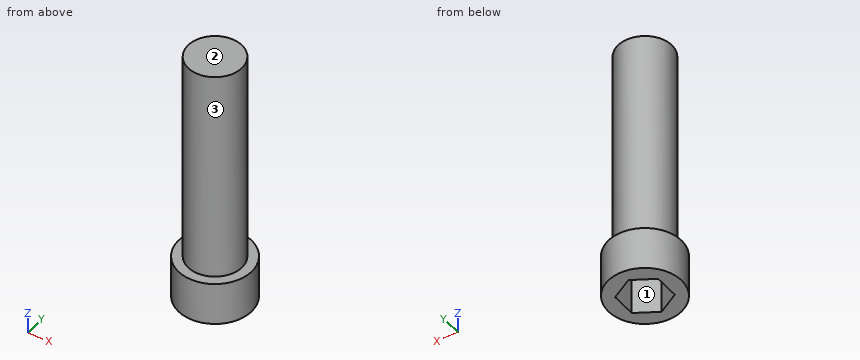
```python
from build123d import *

# Parameters (mm, degrees)
SKETCH1_R           = 1.25
BOSS_EXTRUDE1_DEPTH = 12
SKETCH1_3_R         = 1.7
SKETCH1_3_R_2       = 1.25
BOSS_EXTRUDE2_DEPTH = 2
CUT_EXTRUDE1_DEPTH  = 2


with BuildPart() as part:
    # Sketch1 → Boss-Extrude1 (new body)
    with BuildSketch(Plane.XY):
        Circle(SKETCH1_R)
    extrude(amount=BOSS_EXTRUDE1_DEPTH)

    # Sketch1<3> → Boss-Extrude2 (add)
    with BuildSketch(Plane.XY):
        Circle(SKETCH1_3_R)
        Circle(SKETCH1_3_R_2, mode=Mode.SUBTRACT)
    extrude(amount=BOSS_EXTRUDE2_DEPTH)

    # Sketch3 → Cut-Extrude1 (cut)
    with BuildSketch(Plane(origin=(0, 0, 0), x_dir=(-1, 0, 0), z_dir=(0, 0, -1))):
        Polygon((0.988114182, -0.597464389), (1.01147643, 0.556999789), (0.023362248, 1.154464178), (-0.988114182, 0.597464389), (-1.01147643, -0.556999789), (-0.023362248, -1.154464178), align=None)
    extrude(amount=-CUT_EXTRUDE1_DEPTH, mode=Mode.SUBTRACT)


solid = part.part
```
Can you work these out from the model? Positions are in its coordinate system, mm. Face numbers are marked on the shaded views. Round coordinates to 2 decimals unless told otherwise and drop trailing zeros. Loops run counter-clockwise (first coordinate to the right, second up) from the corner with the lowest first, then second, coordinate; pieces in that order, holes last. Notation, with made-up numbers: (24, 45) -> (41, 45) arc R9 ccw to (41, 61) -> close; hole circle Ø1 at (25, -1). An arc over 180 degrees is marked (long way). One line per item, written item: value. Start each with the question number.
1. If we mould it in two halves opening along Y, with no side actions, what happens to the marked faces 1, 2 and 3? For each: pulls with the +Y half, pulls with the -Y half, needs draft (parallel to the pull), parting line crosses it, or undercut.
2. If I drill on probe 1 along Z at (x, y) = (0.2, 0.75); probe 2 along Z at (x, y) = (-0.95, 1.05); probe 3 along X at (y, z) = (-0.4, 1), over which ranges is the centre line in solid material (lowest first)?
3. If we section it at D-D, the plane z = 5.75: Write out the boundary of the cut face in (x, y).
4. If we section it at B-B, the plane y = 0: Write out the boundary of the cut face in (x, z).
5. For pin 1 (1 mm diameter, centred on x = 1, z = 10, fed in from +Y); pin 2 (2 mm diameter, centred on y = 1, z = 9, fed in from +X), each with a flat end and sliding along its axis, tell me the tip position at first contact or that it passes through.
6. If we section it at A-A, the plane z = 1.5: Write out the boundary of the cut face in (x, y).
7. If we section it at C-C, the plane x = -1.5: Write out the boundary of the cut face in (y, z).
Calculated:
1. face 1: undercut
1. face 2: needs draft
1. face 3: parting line crosses it
2. probe 1: z = 2 to 12
2. probe 2: z = 0 to 2
2. probe 3: x = -1.65 to -0.99, 1.01 to 1.65
3. outline: circle Ø2.5 at (0, 0)
4. outline: (-1.7, 0) -> (-1, 0) -> (-1, 2) -> (1, 2) -> (1, 0) -> (1.7, 0) -> (1.7, 2) -> (1.25, 2) -> (1.25, 12) -> (-1.25, 12) -> (-1.25, 2) -> (-1.7, 2) -> close
5. pin 1: stops at y = 1.15
5. pin 2: stops at x = 1.25
6. outline: circle Ø3.4 at (0, 0); hole (-1.01, 0.56) -> (-0.99, -0.6) -> (0.02, -1.15) -> (1.01, -0.56) -> (0.99, 0.6) -> (-0.02, 1.15) -> close
7. outline: (-0.8, 0) -> (0.8, 0) -> (0.8, 2) -> (-0.8, 2) -> close
